from build123d import *

# Parameters (mm, degrees)
BOSS_EXTRUDE1_DEPTH     = 100
CUT_EXTRUDE3_DEPTH      = 554.165701555
CUT_EXTRUDE3_DEPTH_BACK = 554.165701555
CUT_EXTRUDE5_DEPTH      = 553.962044682
CUT_EXTRUDE5_DEPTH_BACK = 553.962044682
CUT_EXTRUDE7_DEPTH      = 553.962044682
CUT_EXTRUDE7_DEPTH_BACK = 553.962044682
CUT_EXTRUDE9_DEPTH      = 553.962044682
CUT_EXTRUDE9_DEPTH_BACK = 553.962044682


with BuildPart() as part:
    # Sketch1 → Boss-Extrude1 (new body)
    with BuildSketch(Plane.XY):
        with BuildLine():
            ThreePointArc((-192.629438793, 0), (-136.135725272, 33.719619965), (-73.991525193, 55.321722514))
            ThreePointArc((-73.991525193, 55.321722514), (231.264395529, 54.89097703), (535.785554592, 33.719619965))
            ThreePointArc((535.785554592, 33.719619965), (536.798211586, 12.89819156), (539.317827414, -7.795017256))
            ThreePointArc((539.317827414, -7.795017256), (238.042039648, -55.533392614), (-66.568309368, -71.614065728))
            ThreePointArc((-66.568309368, -71.614065728), (-137.800866021, -50.244872094), (-192.629438793, 0))
        make_face()
    extrude(amount=BOSS_EXTRUDE1_DEPTH)

    # Sketch2 → Cut-Extrude3 (cut, two sides: drawn at the far end of the back side and taken through both)
    with BuildSketch(Plane(origin=(0, 0, 0), x_dir=(0, 0, -1), z_dir=(1, 0, 0)).offset(-CUT_EXTRUDE3_DEPTH_BACK)):
        with BuildLine():
            ThreePointArc((-65.447202994, 54.830423707), (-80.892507985, 50.983746932), (-92.956496986, 40.600368972))
            ThreePointArc((-92.956496986, 40.600368972), (-98.736407831, -10.977338679), (-88.967303886, -61.950193259))
            ThreePointArc((-88.967303886, -61.950193259), (-83.10915251, -68.165990231), (-75.589128758, -72.216090516))
            ThreePointArc((-75.589128758, -72.216090516), (-123.822815089, -94.064788666), (-173.378544397, -75.407784602))
            ThreePointArc((-173.378544397, -75.407784602), (-163.802190068, -4.583325871), (-135.262897635, 60.940099743))
            ThreePointArc((-135.262897635, 60.940099743), (-100.366866686, 80.430667917), (-61.326949176, 89.003885783))
            ThreePointArc((-61.326949176, 89.003885783), (-63.560434952, 71.938056418), (-65.447202994, 54.830423707))
        make_face()
    extrude(amount=CUT_EXTRUDE3_DEPTH + CUT_EXTRUDE3_DEPTH_BACK, mode=Mode.SUBTRACT)

    # Sketch3 → Cut-Extrude5 (cut, two sides: drawn at the far end of the back side and taken through both)
    with BuildSketch(Plane(origin=(0, 0, 0), x_dir=(0, 0, -1), z_dir=(1, 0, 0)).offset(-CUT_EXTRUDE5_DEPTH_BACK)):
        with BuildLine():
            ThreePointArc((-74.208303325, 50.886642831), (-50.335012976, 52.211638999), (-26.713093985, 48.511024166))
            ThreePointArc((-26.713093985, 48.511024166), (-16.247111553, 43.841102683), (-7.714956491, 36.189482926))
            ThreePointArc((-7.714956491, 36.189482926), (-2.445034952, -12.786836037), (-8.678058045, -61.649923489))
            ThreePointArc((-8.678058045, -61.649923489), (-17.453523943, -70.69509128), (-29.511303704, -74.360307413))
            ThreePointArc((-29.511303704, -74.360307413), (33.955140221, -79.826327987), (85.286434054, -42.104117568))
            ThreePointArc((85.286434054, -42.104117568), (41.180066923, 16.064388488), (12.319514625, 83.116720583))
            ThreePointArc((12.319514625, 83.116720583), (-170.558095104, 441.821406771), (-74.208303325, 50.886642831))
        make_face()
    extrude(amount=CUT_EXTRUDE5_DEPTH + CUT_EXTRUDE5_DEPTH_BACK, mode=Mode.SUBTRACT)

    # Sketch4 → Cut-Extrude7 (cut, two sides: drawn at the far end of the back side and taken through both)
    with BuildSketch(Plane.XY.offset(-CUT_EXTRUDE7_DEPTH_BACK)):
        Polygon((-79.201401397, 32.882000093), (-79.201401397, -3.122719846), (-222.768125928, 1.814195624), (-233.222282556, 17.110218535), (-80.529357675, 72.456896947), align=None)
    extrude(amount=CUT_EXTRUDE7_DEPTH + CUT_EXTRUDE7_DEPTH_BACK, mode=Mode.SUBTRACT)

    # Sketch7 → Cut-Extrude9 (cut, two sides: drawn at the far end of the back side and taken through both)
    with BuildSketch(Plane.XY.offset(-CUT_EXTRUDE9_DEPTH_BACK)):
        Polygon((-77.622682663, -75.13174066), (-79.880490969, -28.10031394), (-79.880490969, 8.416039234), (-244.452163016, 8.416039234), (-180.732611766, -79.468551396), (-149.591071412, -109.159665737), align=None)
    extrude(amount=CUT_EXTRUDE9_DEPTH + CUT_EXTRUDE9_DEPTH_BACK, mode=Mode.SUBTRACT)


solid = part.part
Design review of the part built by this model. Coordinates are the model's own, in mm. Round coordinates to 2 decimals unless told otherwise and drop trailing zeros. Order: outer loops, then holes, each group sorted by start corner. A loop starts at its lowest first (then second) coordinate and runs counter-clockwise, first axis right, second up.
1) Consider section A-A (x = 41). State the section outline as (y, z) points, plus the area to 3 significant figures.
The answers:
outline: (-69.58, 15.77) arc R25.2 ccw to (-61.65, 8.68) arc R210.93 ccw to (36.19, 7.71) arc R36.96 ccw to (48.51, 26.71) arc R113.61 ccw to (50.89, 74.21) arc R202.65 cw to (49.99, 82.69) arc R34.43 ccw to (40.6, 92.96) arc R173.11 ccw to (-61.95, 88.97) arc R26.72 ccw to (-69.58, 81.08) - close
area: 10,700 mm2
2) For L1, parallel to X at y = 30, z = 6.5; L2, parallel to Z at x = 461, y = 1; L3, parallel to Z at x = 85.5, y = -44.5, list the stretches that pass through material, from the lowest coordinate up.
The answers:
L1: x = -79.2 to 535.86
L2: z = 2.76 to 98.79
L3: z = 5.16 to 94.12
3) Clearance check with flat-ended pins moving along their axes: pin 1 Ø10 at (x, z) = (231.5, 32) entering from +Y; pin 2 Ø11 at (y, z) = (9.5, 71) entering from -X; pin 3 Ø6 at (x, z) = (223, 59.5) entering from -Y. State where each tip first meets the part, or that it passes through.
The answers:
pin 1: stops at y = 50.75
pin 2: stops at x = -79.2
pin 3: stops at y = -57.38
4) Consider section B-B (z = 55). State the section outline as (x, y) points, plus the area to 3 significant figures.
The answers:
outline: (-79.88, -28.1) - (-77.85, -70.48) arc R166.54 ccw to (-66.57, -71.61) arc R2922.96 ccw to (539.32, -7.8) arc R287.33 cw to (535.79, 33.72) arc R4489.88 ccw to (291.56, 52.35) - (-79.85, 52.35) - (-79.2, 32.88) - (-79.2, -3.12) - (-79.88, -3.1) - close
area: 61,600 mm2
5) Consider section D-D (x = 148). State the section outline as (y, z) points.
The answers:
outline: (-63.61, 9.92) arc R25.2 ccw to (-61.65, 8.68) arc R210.93 ccw to (36.19, 7.71) arc R36.96 ccw to (48.51, 26.71) arc R113.61 ccw to (50.89, 74.21) arc R202.65 cw to (49.99, 82.69) arc R34.43 ccw to (40.6, 92.96) arc R173.11 ccw to (-61.95, 88.97) arc R26.72 ccw to (-63.61, 87.75) - close
6) Draft analysis for pull direction Y (two halves, no side actions). For faces 1 (the cylindrical face through (16.3, -66.44, 85.14)), 2 (the flat face through (-79.201, 15, 50)), 3 (the cylindrical face through (225.384, -10.248, 98.763)), 4 (the cylindrical face through (145.994, 43.928, 16.382)), state which applies: released by +Y, released by -Y, zero draft, split by the parting line, or undercut.
The answers:
face 1: released by -Y
face 2: undercut
face 3: split by the parting line
face 4: released by +Y
